from build123d import *

# Parameters (mm, degrees)
SKETCH1_W           = 102
SKETCH1_H           = 96
BOSS_EXTRUDE1_DEPTH = 85
SKETCH3_W           = 90
SKETCH3_H           = 84
CUT_EXTRUDE2_DEPTH  = 80
SKETCH4_W           = 122
SKETCH4_H           = 116
SKETCH4_W_2         = 102
SKETCH4_H_2         = 96
BOSS_EXTRUDE2_DEPTH = 3
SKETCH5_R           = 15
SKETCH5_R_2         = 10
BOSS_EXTRUDE3_DEPTH = 10
CUT_EXTRUDE3_START  = -10
SKETCH8_R           = 10
CUT_EXTRUDE3_DEPTH  = 10
SKETCH9_R           = 1.5
CUT_EXTRUDE4_DEPTH  = 80
SKETCH10_R          = 5
CUT_EXTRUDE_1_DEPTH = 1
FILLET_2_R          = 2


with BuildPart() as part:
    # Sketch1 → Boss-Extrude1 (new body)
    with BuildSketch(Plane(origin=(0, 0, 0), x_dir=(1, 0, 0), z_dir=(0, 1, 0))):
        with Locations((-37.407979351, -6.16081108)):
            Rectangle(SKETCH1_W, SKETCH1_H)
    extrude(amount=BOSS_EXTRUDE1_DEPTH)

    # Sketch3 → Cut-Extrude2 (cut)
    with BuildSketch(Plane(origin=(0, 85, 0), x_dir=(1, 0, 0), z_dir=(0, 1, 0))):
        with Locations((-37.407979351, -6.16081108)):
            Rectangle(SKETCH3_W, SKETCH3_H)
    extrude(amount=-CUT_EXTRUDE2_DEPTH, mode=Mode.SUBTRACT)

    # Sketch4 → Boss-Extrude2 (add)
    with BuildSketch(Plane(origin=(0, 85, 0), x_dir=(1, 0, 0), z_dir=(0, 1, 0))):
        with Locations((-37.407979351, -6.16081108)):
            Rectangle(SKETCH4_W, SKETCH4_H)
        with Locations((-37.407979351, -6.16081108)):
            Rectangle(SKETCH4_W_2, SKETCH4_H_2, mode=Mode.SUBTRACT)
    extrude(amount=-BOSS_EXTRUDE2_DEPTH)

    # Sketch5 → Boss-Extrude3 (add)
    with BuildSketch(Plane(origin=(0, 5, 0), x_dir=(1, 0, 0), z_dir=(0, 1, 0))):
        with Locations(Location((-37.407979351, -6.16081108, 0), (0, 0, 270))):
            Circle(SKETCH5_R)
        with Locations(Location((-37.407979351, -6.16081108, 0), (0, 0, 270))):
            Circle(SKETCH5_R_2, mode=Mode.SUBTRACT)
    extrude(amount=BOSS_EXTRUDE3_DEPTH)

    # Sketch8 → Cut-Extrude3 (cut)
    with BuildSketch(Plane(origin=(0, 5, 0), x_dir=(1, 0, 0), z_dir=(0, 1, 0)).offset(CUT_EXTRUDE3_START)):
        with Locations(Location((-37.407979351, -6.16081108, 0), (0, 0, 270))):
            Circle(SKETCH8_R)
    extrude(amount=CUT_EXTRUDE3_DEPTH, mode=Mode.SUBTRACT)

    # Sketch9 → Cut-Extrude4 (cut)
    with BuildSketch(Plane.ZY.offset(-7.592020649)):
        with Locations(Location((6.16081108, 10, 0), (0, 0, 180))):
            Circle(SKETCH9_R)
    extrude(amount=CUT_EXTRUDE4_DEPTH, mode=Mode.SUBTRACT)

    # Sketch10 → 切除-拉伸1 (cut)
    with BuildSketch(Plane(origin=(0, 5, 0), x_dir=(1, 0, 0), z_dir=(0, 1, 0))):
        with Locations(Location((-2.407979351, 26.487445273, 0), (0, 0, 270))):
            Circle(SKETCH10_R)
        with Locations(Location((-2.407979351, -38.827477746, 0), (0, 0, 270))):
            Circle(SKETCH10_R)
        with Locations(Location((-72.407979351, -38.827477746, 0), (0, 0, 270))):
            Circle(SKETCH10_R)
        with Locations(Location((-72.407979351, 26.487445273, 0), (0, 0, 270))):
            Circle(SKETCH10_R)
    extrude(amount=-CUT_EXTRUDE_1_DEPTH, mode=Mode.SUBTRACT)

    # 圆角2
    fillet_2_edges = [part.edges().sort_by_distance(p)[0] for p in [
        (-37.407979351, 85, -35.83918892),
        (-82.407979351, 85, 6.16081108),
        (-37.407979351, 85, 48.16081108),
        (7.592020649, 85, 6.16081108),
    ]]
    fillet(fillet_2_edges, radius=FILLET_2_R)


solid = part.part
The listing builds one solid part. Answer for the finished solid, in the listing's coordinates (mm). A direction names the side the tool comes from. Give positions to 0.01 mm unless a question says otherwise; leave off trailing zeros. Loops run counter-clockwise (first coordinate to the right, second up) from the corner with the lowest first, then second, coordinate; pieces in that order, holes last. Notation, with made-up numbers: (2, 29) - (21, 29) arc R19 cw to (21, 37) - close; hole circle Ø2 at (40, 22). An arc over 180 degrees is marked (long way). Use one line per item in the form item = value.
1. Section A-A on z = 9.5 is taken. Give the vertices of the cut face in (x, y), then the cut area to 3 significant figures.
Calculated:
outline = (-98.41, 82) - (-88.41, 82) - (-88.41, 0) - (-46.83, 0) - (-46.83, 15) - (-52.03, 15) - (-52.03, 5) - (-82.41, 5) - (-82.41, 83) arc R2 ccw to (-84.41, 85) - (-98.41, 85) - close; (-27.98, 0) - (13.59, 0) - (13.59, 82) - (23.59, 82) - (23.59, 85) - (9.59, 85) arc R2 ccw to (7.59, 83) - (7.59, 5) - (-22.78, 5) - (-22.78, 15) - (-27.98, 15) - close
area = 1,540 mm^2
2. Find the intervals of material crossed by line 1 along X through (y, z) = (72, 5); line 2 along Z through (x, y) = (-50, 10); line 3 along Z through (x, y) = (-19.5, 27), in increasing order. Write a range as [from, to].
Calculated:
line_1 = [-88.41, -82.41], [7.59, 13.59]
line_2 = [-41.84, -35.84], [-1.99, 4.66], [7.66, 14.31], [48.16, 54.16]
line_3 = [-41.84, -35.84], [48.16, 54.16]
3. The mould has two halves that part along X. Classify faces 5 (the face through (13.592, 40, 7)), 6 (the face through (-38, 85, 57)), 7 (the face through (-38, 45, 48.161)): pulls with the +X half, pulls with the -X half, needs draft (parallel to the pull), parting line crosses it, or undercut.
Calculated:
face_5 = pulls with the +X half
face_6 = needs draft
face_7 = undercut
4. Section C-C on z = 24 is taken. Give the vertices of the cut face in (x, y).
Calculated:
outline = (-98.41, 82) - (-88.41, 82) - (-88.41, 0) - (13.59, 0) - (13.59, 82) - (23.59, 82) - (23.59, 85) - (9.59, 85) arc R2 ccw to (7.59, 83) - (7.59, 5) - (-82.41, 5) - (-82.41, 83) arc R2 ccw to (-84.41, 85) - (-98.41, 85) - close
5. Given pin 1 Ø8 at (x, y) = (-48, 65) entering from -Z; pin 2 Ø8 at (x, y) = (-84.5, 64.5) entering from +Z; pin 3 Ø11 at (x, z) = (-2, 38) entering from +Y, each flat-ended and moving along its own axis, determine where each tip first touches the part or whether it passes through.
Calculated:
pin_1 = -41.84
pin_2 = 54.16
pin_3 = 5
6. Section B-B on y = 54 is taken. Give the vertices of the cut face in (x, z).
Calculated:
outline = (-88.41, -41.84) - (13.59, -41.84) - (13.59, 54.16) - (-88.41, 54.16) - close; hole (-82.41, -35.84) - (7.59, -35.84) - (7.59, 48.16) - (-82.41, 48.16) - close
7. Section D-D on x = -50.5 is taken. Give the vertices of the cut face in (y, z), then the cut area to 3 significant figures.
Calculated:
outline = (0, -41.84) - (82, -41.84) - (82, -51.84) - (85, -51.84) - (85, -37.84) arc R2 ccw to (83, -35.84) - (5, -35.84) - (5, -1.16) - (15, -1.16) - (15, 13.48) - (5, 13.48) - (5, 48.16) - (83, 48.16) arc R2 ccw to (85, 50.16) - (85, 64.16) - (82, 64.16) - (82, 54.16) - (0, 54.16) - close; hole circle Ø3 at (10, 6.16)
area = 1,640 mm^2
8. Which of the six approach directions +Z, -Z, +X, -X, +Y, -Y give full straight-line access (tool end or side, diameter ignored) to faces 1 (the face through (-72, 4, 39)), 2 (the face through (-24.93, 11.33, 5.47)), 3 (the face through (-38, 40, -41.839)), 4 (the face through (-38, 0, -5))?
Calculated:
face_1 = +Y
face_2 = none
face_3 = -Z, +X, -X, -Y
face_4 = +Z, -Z, +X, -X, -Y
